from build123d import *
from OCP.BRepFilletAPI import BRepFilletAPI_MakeChamfer

# Parameters (mm, degrees)
SKETCH1_W           = 60
SKETCH1_H           = 45
BOSS_EXTRUDE1_DEPTH = 30
SKETCH2_W           = 6.5
SKETCH2_H           = 16
CUT_EXTRUDE1_DEPTH  = 20
CHAMFER1_SIZE       = 5
CHAMFER1_SIZE2      = 0.437443318
CHAMFER2_SIZE       = 5
CHAMFER2_SIZE2      = 5.958767963
CUT_EXTRUDE2_DEPTH  = 10
CHAMFER3_SIZE       = 3
CHAMFER3_SIZE2      = 2


with BuildPart() as part:
    # Sketch1 → Boss-Extrude1 (new body)
    with BuildSketch(Plane(origin=(0, 0, 0), x_dir=(1, 0, 0), z_dir=(0, 1, 0))):
        with Locations((-30, 22.5)):
            Rectangle(SKETCH1_W, SKETCH1_H)
    extrude(amount=BOSS_EXTRUDE1_DEPTH)

    # Sketch2 → Cut-Extrude1 (cut)
    with BuildSketch(Plane(origin=(0, 0, 0), x_dir=(-1, 0, 0), z_dir=(0, -1, 0))):
        with Locations((47.75, 21)):
            Rectangle(SKETCH2_W, SKETCH2_H)
        with Locations((12.75, 21)):
            Rectangle(SKETCH2_W, SKETCH2_H)
    extrude(amount=-CUT_EXTRUDE1_DEPTH, mode=Mode.SUBTRACT)

    # Chamfer1: one chamfer whose edges measure the first distance from different faces: ONE call of the kernel's chamfer builder (chamfer() names one face for all edges)
    chamfer1_edges_1 = [part.edges().sort_by_distance(p)[0] for p in [
        (-51, 20, -21),
    ]]
    chamfer1_side_1 = [part.faces().sort_by_distance(p)[0] for p in [
        (-51, 10, -21),
    ]]
    chamfer1_edges_2 = [part.edges().sort_by_distance(p)[0] for p in [
        (-44.5, 20, -21),
    ]]
    chamfer1_side_2 = [part.faces().sort_by_distance(p)[0] for p in [
        (-44.5, 10, -21),
    ]]
    chamfer1_edges_3 = [part.edges().sort_by_distance(p)[0] for p in [
        (-16, 20, -21),
    ]]
    chamfer1_side_3 = [part.faces().sort_by_distance(p)[0] for p in [
        (-16, 10, -21),
    ]]
    chamfer1_edges_4 = [part.edges().sort_by_distance(p)[0] for p in [
        (-9.5, 20, -21),
    ]]
    chamfer1_side_4 = [part.faces().sort_by_distance(p)[0] for p in [
        (-9.5, 10, -21),
    ]]
    chamfer1 = BRepFilletAPI_MakeChamfer(part.part.solid().wrapped)
    for e in chamfer1_edges_1:
        chamfer1.Add(CHAMFER1_SIZE, CHAMFER1_SIZE2, e.wrapped, chamfer1_side_1[0].wrapped)  # the first distance lies on this face
    for e in chamfer1_edges_2:
        chamfer1.Add(CHAMFER1_SIZE, CHAMFER1_SIZE2, e.wrapped, chamfer1_side_2[0].wrapped)  # the first distance lies on this face
    for e in chamfer1_edges_3:
        chamfer1.Add(CHAMFER1_SIZE, CHAMFER1_SIZE2, e.wrapped, chamfer1_side_3[0].wrapped)  # the first distance lies on this face
    for e in chamfer1_edges_4:
        chamfer1.Add(CHAMFER1_SIZE, CHAMFER1_SIZE2, e.wrapped, chamfer1_side_4[0].wrapped)  # the first distance lies on this face
    add(Compound.cast(chamfer1.Shape()), mode=Mode.REPLACE)

    # Chamfer2: one chamfer whose edges measure the first distance from different faces: ONE call of the kernel's chamfer builder (chamfer() names one face for all edges)
    chamfer2_edges_1 = [part.edges().sort_by_distance(p)[0] for p in [
        (-47.75, 20, -29),
    ]]
    chamfer2_side_1 = [part.faces().sort_by_distance(p)[0] for p in [
        (-47.75, 9.857394508, -29),
    ]]
    chamfer2_edges_2 = [part.edges().sort_by_distance(p)[0] for p in [
        (-12.75, 20, -29),
    ]]
    chamfer2_side_2 = [part.faces().sort_by_distance(p)[0] for p in [
        (-12.75, 9.857394508, -29),
    ]]
    chamfer2_edges_3 = [part.edges().sort_by_distance(p)[0] for p in [
        (-12.75, 20, -13),
    ]]
    chamfer2_side_3 = [part.faces().sort_by_distance(p)[0] for p in [
        (-12.75, 9.857394508, -13),
    ]]
    chamfer2_edges_4 = [part.edges().sort_by_distance(p)[0] for p in [
        (-47.75, 20, -13),
    ]]
    chamfer2_side_4 = [part.faces().sort_by_distance(p)[0] for p in [
        (-47.75, 9.857394508, -13),
    ]]
    chamfer2 = BRepFilletAPI_MakeChamfer(part.part.solid().wrapped)
    for e in chamfer2_edges_1:
        chamfer2.Add(CHAMFER2_SIZE, CHAMFER2_SIZE2, e.wrapped, chamfer2_side_1[0].wrapped)  # the first distance lies on this face
    for e in chamfer2_edges_2:
        chamfer2.Add(CHAMFER2_SIZE, CHAMFER2_SIZE2, e.wrapped, chamfer2_side_2[0].wrapped)  # the first distance lies on this face
    for e in chamfer2_edges_3:
        chamfer2.Add(CHAMFER2_SIZE, CHAMFER2_SIZE2, e.wrapped, chamfer2_side_3[0].wrapped)  # the first distance lies on this face
    for e in chamfer2_edges_4:
        chamfer2.Add(CHAMFER2_SIZE, CHAMFER2_SIZE2, e.wrapped, chamfer2_side_4[0].wrapped)  # the first distance lies on this face
    add(Compound.cast(chamfer2.Shape()), mode=Mode.REPLACE)

    # Sketch4 → Cut-Extrude2 (cut)
    with BuildSketch(Plane(origin=(0, 0, -45), x_dir=(-1, 0, 0), z_dir=(0, 0, -1))):
        with BuildLine():
            Line((12.7, 0), (29.5, 0))
            ThreePointArc((29.5, 0), (35.280602383, 6.276082414), (43.81191296, 6.13008847))
            ThreePointArc((43.81191296, 6.13008847), (48.288831578, 7.478397416), (47.430644896, 12.074510224))
            ThreePointArc((47.430644896, 12.074510224), (26.808734298, 15.404376803), (12.7, 0))
        make_face()
    extrude(amount=-CUT_EXTRUDE2_DEPTH, mode=Mode.SUBTRACT)

    # Chamfer3
    chamfer3_edges = [part.edges().sort_by_distance(p)[0] for p in [
        (-51, 0, -21),
        (-47.75, 0, -29),
        (-44.5, 0, -21),
        (-47.75, 0, -13),
        (-16, 0, -21),
        (-12.75, 0, -29),
        (-9.5, 0, -21),
        (-12.75, 0, -13),
    ]]
    chamfer3_side = [part.faces().sort_by_distance(p)[0] for p in [
        (-30.620998279, 0, -21.36919105),
    ]]
    chamfer(chamfer3_edges, length=CHAMFER3_SIZE, length2=CHAMFER3_SIZE2, reference=chamfer3_side[0])


solid = part.part
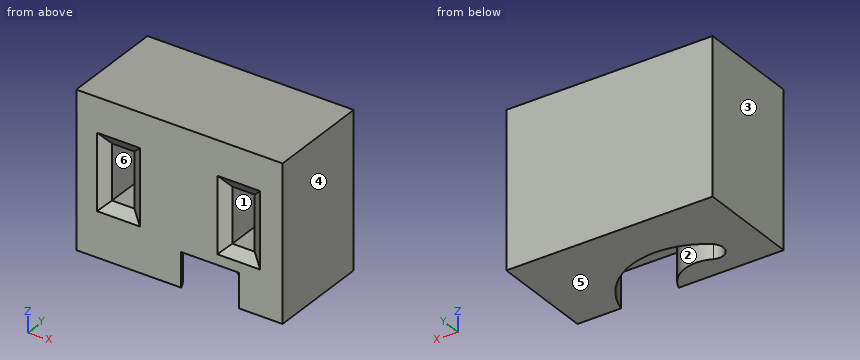
Geometry check sheet. Reference: the model listing, model coordinates, mm. Face numbers are marked on the shaded views. A direction names the side the tool comes from. Round coordinates to 2 decimals unless told otherwise and drop trailing zeros. Loops run counter-clockwise (first coordinate to the right, second up) from the corner with the lowest first, then second, coordinate; pieces in that order, holes last.
Item 1: Cross-section at D-D on z = -17. Record the boundary of the cut face in (x, y).
Item 2: Mould release check, pull along X, two halves, no side actions. Record for the marked faces 1, 2, 3 and 4: pulls with the +X half, pulls with the -X half, needs draft (parallel to the pull), parting line crosses it, or undercut.
Item 3: Cross-section at C-C on x = -14.5. Record the boundary of the cut face in (y, z).
Item 4: Cross-section at A-A on z = -22. Record the boundary of the cut face in (x, y).
Item 5: Access from +Z, -Z, +X, -X, +Y, -Y to the whole of each face (thin tool, end or side, straight path). Record for the marked faces 5 and 6.
Item 6: Cross-section at B-B on y = 19.25. Record the boundary of the cut face in (x, z), then the cut area to 3 significant figures.
Item 7: Gauge pin test, flat ends, axial feed: pin 1 (3.5 mm diameter, centred on x = -12, z = -20.5, fed in from -Y); pin 2 (4 mm diameter, centred on x = -27, y = 4.5, fed in from -Z); pin 3 (4.5 mm diameter, centred on x = -47.5, z = -20.5, fed in from -Y). Record the tip position at first contact, or that the pin passes through.
Item 8: Thickness scan on line 1 (X direction, y = 11.5, z = -25); line 2 (X direction, y = 18, z = -17); line 3 (Y direction, x = -32.5, z = -39.5). Record the ranges inside material, lowest first.
Answer sheet:
1. outline: (-60, 0) - (-54, 0) - (-51, 2) - (-51, 15) - (-50.71, 18.36) - (-44.79, 18.36) - (-44.5, 15) - (-44.5, 2) - (-41.5, 0) - (-19, 0) - (-16, 2) - (-16, 15) - (-15.71, 18.36) - (-9.79, 18.36) - (-9.5, 15) - (-9.5, 2) - (-6.5, 0) - (0, 0) - (0, 30) - (-60, 30) - close
2. face 1: undercut
2. face 2: undercut
2. face 3: pulls with the -X half
2. face 4: pulls with the +X half
3. outline: (0, -35) - (4.75, -35) - (4.75, -45) - (30, -45) - (30, 0) - (0, 0) - (0, -10) - (2, -13) - (15, -13) - (20, -18.96) - (20, -23.04) - (15, -29) - (2, -29) - (0, -32) - close
4. outline: (-60, 0) - (-54, 0) - (-51, 2) - (-51, 15) - (-50.56, 20) - (-44.94, 20) - (-44.5, 15) - (-44.5, 2) - (-41.5, 0) - (-19, 0) - (-16, 2) - (-16, 15) - (-15.56, 20) - (-9.94, 20) - (-9.5, 15) - (-9.5, 2) - (-6.5, 0) - (0, 0) - (0, 30) - (-60, 30) - close
5. face 5: -Z, +X, -X, +Y, -Y
5. face 6: -Y
6. outline: (-60, -45) - (0, -45) - (0, 0) - (-60, 0) - close; hole (-50.63, -23.94) - (-44.87, -23.94) - (-44.87, -18.06) - (-50.63, -18.06) - close; hole (-15.63, -23.94) - (-9.87, -23.94) - (-9.87, -18.06) - (-15.63, -18.06) - close
6. area: 2,630 mm2
7. pin 1: stops at y = 19.82
7. pin 2: stops at z = -35
7. pin 3: stops at y = 19.41
8. line 1: x = -60 to -51, -44.5 to -16, -9.5 to 0
8. line 2: x = -60 to -50.74, -44.76 to -15.74, -9.76 to 0
8. line 3: y = 0 to 4.52, 16.57 to 30
